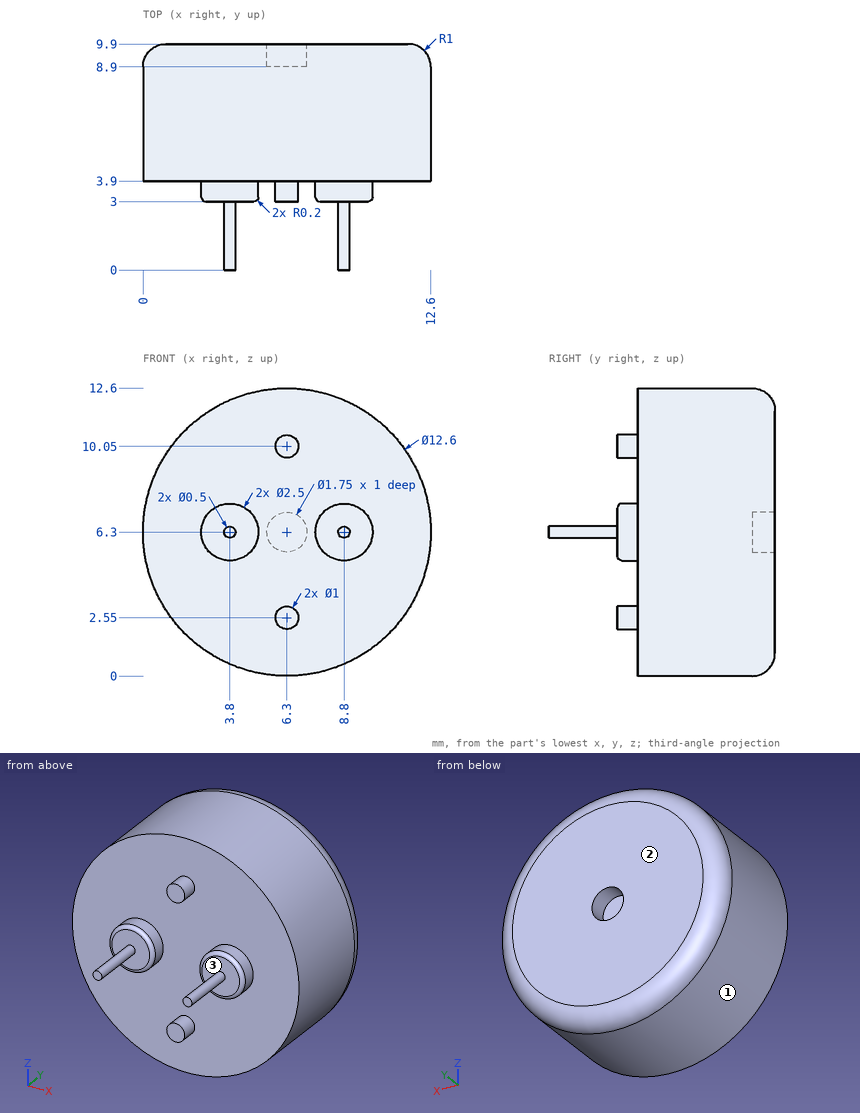
Print and shaded views of the part. All mm, measured from the part's lowest x, y and z. Coordinates: 2 decimals unless noted, no trailing zeros. Write item = value, one per line. Start each with the question number.
Item 1: Drop flat-ended pins along their axis: pin 1 Ø5 at (x, z) = (6, 1.5) entering from -Y; pin 2 Ø1.4 at (x, z) = (6.3, 6.3) entering from -Y; pin 3 Ø0.9 at (x, z) = (6.5, 6) entering from +Y. Give the stop position or say it passes through.
Item 2: Pull direction X, two halves, no side cores. Call the marked faces 1, 2 and 3: +X half, -X half, draft (parallel to the pull), parting line (faces both ways), or undercut.
Item 3: Wall check: probe 1 along Y at (x, z) = (2.5, 3.25); probe 2 along Y at (x, z) = (6.25, 9.75); probe 3 along X at (y, z) = (9.7, 6.3) (1 decimal). Give the ranges that are in metal, low to high. Write a range as [from, to].
Answers:
q1.pin_1 = 3
q1.pin_2 = 3.9
q1.pin_3 = 8.9
q2.face_1 = parting line
q2.face_2 = draft
q2.face_3 = undercut
q3.probe_1 = [3.9, 9.9]
q3.probe_2 = [3, 9.9]
q3.probe_3 = [0.4, 5.4], [7.2, 12.2]
